```python
from build123d import *

# Parameters (mm, degrees)
BOX012_W          = 66
BOX012_H          = 3
BOX012_DEPTH      = 5
FILLET003_R       = 4
CYLINDER014_R     = 1
CYLINDER014_DEPTH = 10
BOX013_W          = 8
BOX013_H          = 9
BOX013_DEPTH      = 3.5
FILLET002_R       = 3
ARRAY011_X_COUNT  = 2
ARRAY011_X_PITCH  = 58


with BuildPart() as long_cube_fillet:
    # Box012 → Box012 (new body)
    with BuildSketch(Plane.XY):
        with Locations((33, 1.5)):
            Rectangle(BOX012_W, BOX012_H)
    extrude(amount=BOX012_DEPTH)

    # Fillet003
    fillet003_edges = [long_cube_fillet.edges().sort_by_distance(p)[0] for p in [
        (0, 1.5, 5),
        (66, 1.5, 5),
    ]]
    fillet(fillet003_edges, radius=FILLET003_R)


with BuildPart() as cylinder002:
    # Cylinder014 → Cylinder014 (new body)
    with BuildSketch(Plane(origin=(4, 3, -5), x_dir=(1, 0, 0), z_dir=(0, 0, 1))):
        Circle(CYLINDER014_R)
    extrude(amount=CYLINDER014_DEPTH)


with BuildPart() as obj1:
    # Box013 → Box013 (new body)
    with BuildSketch(Plane.XY.offset(-3.5)):
        with Locations((4, 4.5)):
            Rectangle(BOX013_W, BOX013_H)
    extrude(amount=BOX013_DEPTH)

    # Fillet002
    fillet002_edges = [obj1.edges().sort_by_distance(p)[0] for p in [
        (0, 0, -1.75),
        (8, 0, -1.75),
    ]]
    fillet(fillet002_edges, radius=FILLET002_R)

    # Cut008: cut Cylinder002
    add(cylinder002.part, mode=Mode.SUBTRACT)

    # Array011 X: obj1_2


with BuildPart() as obj1_1:
    add(obj1.part)
    with Locations(*[(i * ARRAY011_X_PITCH, 0, 0) for i in range(1, ARRAY011_X_COUNT)]):
        add(obj1.part)


with BuildPart() as obj1_2:
    # Array011 placement: moved
    add(obj1_1.part.moved(Location((0, -6, 0))))

    # Fusion007: union long cube fillet
    add(long_cube_fillet.part)


solid = obj1_2.part
```
Design review of the part built by this model. Coordinates are the model's own, in mm. A direction names the side the tool comes from. Round coordinates to 2 decimals unless told otherwise and drop trailing zeros. Order: outer loops, then holes, each group sorted by start corner. A loop starts at its lowest first (then second) coordinate and runs counter-clockwise, first axis right, second up. Notation, with made-up numbers: (67, 63.25) - (124, 63.25) arc R21 cw to (124, 77.25) - close; hole circle Ø4 at (-2.5, 89.5). An arc over 180 degrees is marked (long way). Return JSON: item names as keys, results as strings.
Q1. For pin 1 Ø3 at (x, y) = (63, -2) entering from +Z; pin 2 Ø1 at (x, z) = (48.5, 2) entering from -Y; pin 3 Ø2.5 at (x, y) = (31, 2) entering from -Z, all flat-tipped, find the tip position at first contact; note any pin that passes through.
Computed values:
{"pin 1": "stops at z = 0", "pin 2": "stops at y = 0", "pin 3": "stops at z = 0"}
Q2. Machinability: for faces 1 (the flat face through (33, 0, 2)), 2 (the flat face through (62, -6, -2)), 3 (the flat face through (58, 0, -2)), 4 (the cylindrical face through (7.1, -5.14, -1.73)), which of the approach directions +Z, -Z, +X, -X, +Y, -Y give a long, thin tool a straight path to every point of the face, cutting with its end or side? Answer none if there is none.
Computed values:
{"face 1": "+Z, +X, -X, -Y", "face 2": "+Z, -Z, +X, -X, -Y", "face 3": "-Z, +Y, -Y", "face 4": "+Z, -Z, -Y"}
Q3. Consider section A-A on y = -0.75. Write out the cut boundary in (x, z).
Computed values:
{"outline": "(0, -3.5) - (8, -3.5) - (8, 0) - (0, 0) - close; (58, -3.5) - (66, -3.5) - (66, 0) - (58, 0) - close"}
Q4. Consider section C-C on z = 3.5. Write out the cut boundary in (x, y).
Computed values:
{"outline": "(0.88, 0) - (65.12, 0) - (65.12, 3) - (0.88, 3) - close"}
Q5. Consider section D-D on x = 60. Write out the cut boundary in (y, z), plus the area to 3 significant figures.
Computed values:
{"outline": "(-5.83, -3.5) - (3, -3.5) - (3, 5) - (0, 5) - (0, 0) - (-5.83, 0) - close", "area": "45.9 mm2"}
Q6. Wall thickness on L1, parallel to X at y = -3, z = -2.3; L2, parallel to Y at x = 62, z = -2; L3, parallel to X at y = -3.5, z = -0.5: over which ranges is each line inside the solid? List them lowest first. Write a range as [from, to].
Computed values:
{"L1": "x = [0, 3], [5, 8], [58, 61], [63, 66]", "L2": "y = [-6, -4], [-2, 3]", "L3": "x = [0.04, 3.13], [4.87, 7.96], [58.04, 61.13], [62.87, 65.96]"}
Q7. The part is to be moulded in two halves that separate along Y. For faces 5 (the cylindrical face through (61, -3, -2)), 6 (the cylindrical face through (3, -3, -2)), 7 (the flat face through (33, 2, 0)), 8 (the cylindrical face through (65.1, -5.14, -1.73)), say which applies: pulls with the +Y half, pulls with the -Y half, needs draft (parallel to the pull), parting line crosses it, or undercut.
Computed values:
{"face 5": "undercut", "face 6": "undercut", "face 7": "needs draft", "face 8": "pulls with the -Y half"}
Q8. Consider section B-B on x = 42. Write out the cut boundary in (y, z), plus the area to 3 significant figures.
Computed values:
{"outline": "(0, 0) - (3, 0) - (3, 5) - (0, 5) - close", "area": "15.0 mm2"}
